Geometry check sheet. Reference: drawing and pictorial views, mm from the part's lowest x, y, z. A direction names the side the tool comes from. Coordinates: 2 decimals unless noted, no trailing zeros. Write each loop counter-clockwise with the first axis right and the second up, starting at its lowest first coordinate (ties: lowest second). Pieces come first, ordered by that corner, then holes.
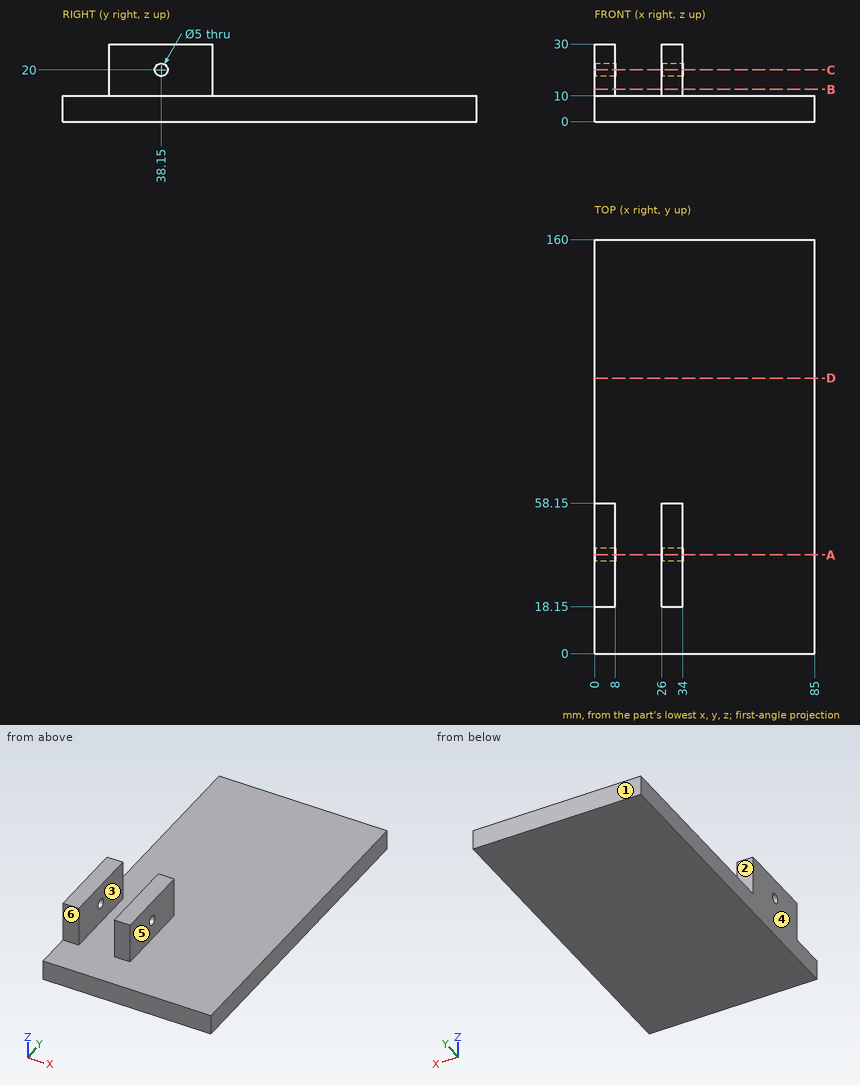
1. Sectioned sample at B-B, the plane z = 12.5. Record the boundary of the cut face in (x, y), and give its area (3 significant figures).
2. Gauge pin test, flat ends, axial feed: P1, Ø4, axis at y = 38.15, z = 20, coming from the -X side; P2, Ø3, axis at y = 48.5, z = 17.5, coming from the +X side; P3, Ø2.5, axis at x = 2.5, z = 17, coming from the -Y side; P4, Ø6, axis at x = 10, z = 27, coming from the +Y side. Record the tip position at first contact, or that the pin passes through.
3. Draft check along X on the marked faces 3, 4, 5 and 6. Enter one of: pulls with the +X half, pulls with the -X half, needs draft (parallel to the pull), parting line crosses it, or undercut.
4. Sectioned sample at C-C, the plane z = 20. Record the boundary of the cut face in (x, y), and give its area (3 significant figures).
5. Tool access check on the marked faces 1 and 2. Record the directions out of +Z, -Z, +X, -X, +Y, -Y that give a thin tool (end or side, any length) a straight path to the whole face; none if there is none.
6. Material ranges on L1, parallel to Y at x = 28, z = 20; L2, parallel to X at y = 57, z = 11; L3, parallel to Z at x = 28, y = 38, recorded low to high.
7. Sectioned sample at A-A, the plane y = 38.15. Record the boundary of the cut face in (x, z).
8. Sectioned sample at D-D, the plane y = 106.5. Record the boundary of the cut face in (x, z).
Outcome:
1. outline: (0, 18.15) - (8, 18.15) - (8, 58.15) - (0, 58.15) - close; (26, 18.15) - (34, 18.15) - (34, 58.15) - (26, 58.15) - close
1. area: 640 mm2
2. P1: passes through
2. P2: stops at x = 34
2. P3: stops at y = 18.15
2. P4: stops at y = 58.15
3. face 3: undercut
3. face 4: pulls with the -X half
3. face 5: pulls with the +X half
3. face 6: needs draft
4. outline: (0, 18.15) - (8, 18.15) - (8, 35.65) - (0, 35.65) - close; (0, 40.65) - (8, 40.65) - (8, 58.15) - (0, 58.15) - close; (26, 18.15) - (34, 18.15) - (34, 35.65) - (26, 35.65) - close; (26, 40.65) - (34, 40.65) - (34, 58.15) - (26, 58.15) - close
4. area: 560 mm2
5. face 1: +Z, -Z, +X, -X, +Y
5. face 2: +Z, +X, -X, +Y
6. L1: y = 18.15 to 35.65, 40.65 to 58.15
6. L2: x = 0 to 8, 26 to 34
6. L3: z = 0 to 17.5, 22.5 to 30
7. outline: (0, 0) - (85, 0) - (85, 10) - (34, 10) - (34, 17.5) - (26, 17.5) - (26, 10) - (8, 10) - (8, 17.5) - (0, 17.5) - close; (0, 22.5) - (8, 22.5) - (8, 30) - (0, 30) - close; (26, 22.5) - (34, 22.5) - (34, 30) - (26, 30) - close
8. outline: (0, 0) - (85, 0) - (85, 10) - (0, 10) - close
